Build history of the part. All positions in model axes, mm. Coordinates: 2 decimals unless noted, no trailing zeros. Order: outer loops, then holes, each group sorted by start corner. A loop starts at its lowest first (then second) coordinate and runs counter-clockwise, first axis right, second up. Notation, with made-up numbers: (-13.5, 59) - (-2.5, 59) arc R20 cw to (-2.5, 84) - close; hole circle Ø5 at (-3.75, 84). An arc over 180 degrees is marked (long way). One line per item, written item: value.
from build123d import *

# Parameters (mm, degrees)
SKETCH1_W                                       = 12.7
SKETCH1_H                                       = 9.525
BOSS_EXTRUDE1_DEPTH                             = 3.175
CSK_FOR_M3_FLAT_HEAD_MACHINE_SCREW1_D           = 3.4
CSK_FOR_M3_FLAT_HEAD_MACHINE_SCREW1_CSINK_D     = 6.3
CSK_FOR_M3_FLAT_HEAD_MACHINE_SCREW1_CSINK_ANGLE = 90
FILLET1_R                                       = 2.54


with BuildPart() as part:
    # Sketch1 → Boss-Extrude1 (new body)
    with BuildSketch(Plane(origin=(0, 0, 0), x_dir=(1, 0, 0), z_dir=(0, 1, 0))):
        Rectangle(SKETCH1_W, SKETCH1_H)
    extrude(amount=BOSS_EXTRUDE1_DEPTH)

    # CSK for M3 Flat Head Machine Screw1 (through all)
    with Locations(Plane(origin=(0, 3.175, 0), x_dir=(1, 0, 0), z_dir=(0, 1, 0))):
        with Locations((-1.5875, 0)):
            CounterSinkHole(CSK_FOR_M3_FLAT_HEAD_MACHINE_SCREW1_D / 2, CSK_FOR_M3_FLAT_HEAD_MACHINE_SCREW1_CSINK_D / 2, counter_sink_angle=CSK_FOR_M3_FLAT_HEAD_MACHINE_SCREW1_CSINK_ANGLE)

    # Fillet1
    fillet1_edges = [part.edges().sort_by_distance(p)[0] for p in [
        (6.35, 1.5875, -4.7625),
        (6.35, 1.5875, 4.7625),
    ]]
    fillet(fillet1_edges, radius=FILLET1_R)


solid = part.part
1. Flat gauge pin, fed straight in: P1, Ø4.5, axis at x = -1.59, z = 0, coming from the +Y side. Where does the tip first touch, or does it go through?
Values found:
P1: stops at y = 2.28
2. Band-saw the part on D-D, the plane z = 4. Give the cut face in (x, y) (3 decimals), and give its area (3 significant figures).
Values found:
outline: (-6.35, 0) - (5.624, 0) - (5.624, 3.175) - (-6.35, 3.175) - close
area: 38.0 mm2
3. Two-plate mould, pull along Z, no slides. Class faces 1 (the face through (0, 0, -1)), 2 (the face through (-1, 2, -4.762)), 3 (the face through (-2.37, 0.85, 1.51)), 4 (the face through (5.626, 1.61, 3.999)): pulls with the +Z half, pulls with the -Z half, needs draft (parallel to the pull), parting line crosses it, or undercut.
Values found:
face 1: needs draft
face 2: pulls with the -Z half
face 3: undercut
face 4: pulls with the +Z half
4. Band-saw the part on A-A, the plane y = 0.35. Give the cut face in (x, z), and give its area (3 significant figures).
Values found:
outline: (-6.35, -4.76) - (3.81, -4.76) arc R2.54 ccw to (6.35, -2.22) - (6.35, 2.22) arc R2.54 ccw to (3.81, 4.76) - (-6.35, 4.76) - close; hole circle Ø3.4 at (-1.59, 0)
area: 109 mm2
5. Probe line 1 along X through (y, z) = (1.95, 0.75); line 2 along Z through (x, y) = (0.5, 2.85); line 3 along X through (y, z) = (2.9, -1.25). List the from-to ranges inside material, lowest first.
Values found:
line 1: x = -6.35 to -3.36, 0.19 to 6.35
line 2: z = -4.76 to -1.9, 1.9 to 4.76
line 3: x = -6.35 to -4.18, 1 to 6.35
